from build123d import *

# Parameters (mm, degrees)
F0_R     = 6.35
F0_R_2   = 14.2875
F1_DEPTH = 12.7


with BuildPart() as f1:
    # F0 (on Top) → F1 (new body)
    with BuildSketch(Plane.XY):
        Polygon((-367.050953, -215.623875), (-273.490369, -377.910882), (158.309631, -377.910882), (251.870214, -215.623875), (36.072131, 158.384718), (-151.252869, 158.384718), align=None)
        with Locations((-258.135842, -333.942033)):
            Circle(F0_R, mode=Mode.SUBTRACT)
        with Locations((-289.851294, -278.929488)):
            Circle(F0_R_2, mode=Mode.SUBTRACT)
        with Locations((-321.566746, -223.916943)):
            Circle(F0_R, mode=Mode.SUBTRACT)
        with Locations((142.955103, -333.942033)):
            Circle(F0_R, mode=Mode.SUBTRACT)
        with Locations((174.670555, -278.929488)):
            Circle(F0_R_2, mode=Mode.SUBTRACT)
        with Locations((205.089922, -226.165088)):
            Circle(F0_R, mode=Mode.SUBTRACT)
        with Locations((-121.090369, 122.945368)):
            Circle(F0_R, mode=Mode.SUBTRACT)
        with Locations((-57.590369, 122.945368)):
            Circle(F0_R_2, mode=Mode.SUBTRACT)
        with Locations((5.909631, 122.945368)):
            Circle(F0_R, mode=Mode.SUBTRACT)
    extrude(amount=F1_DEPTH)


solid = f1.part
Source: CAD feature listing. Evaluate the final solid. Frame: model axes, mm. Round coordinates to 2 decimals unless told otherwise and drop trailing zeros. Loops run counter-clockwise (first coordinate to the right, second up) from the corner with the lowest first, then second, coordinate; pieces in that order, holes last. Notation, with made-up numbers: M 21.25,63.25 L 51.25,63.25 A7 ccw 51.25,75.25 Z; hole C 65,-35.5 d2. An arc over 180 degrees is marked long. Answer as CSV lines item,"result".
Q1. Cut plane C-C (y = -49). Return the cut outline in (x, z), plus the area to 3 significant figures.
Verdict:
outline,"M -270.91,0 L 155.73,0 L 155.73,12.7 L -270.91,12.7 Z"
area,"5,420 mm^2"
Q2. Cut plane B-B (x = 52.5). Return the cut outline in (y, z), plus the area to 3 significant figures.
Verdict:
outline,"M -377.91,0 L 129.91,0 L 129.91,12.7 L -377.91,12.7 Z"
area,"6,450 mm^2"
Q3. Cut plane A-A (z = 5.25). Count the separate pieces of the cut face and the enclosed holes in it, plus the area to 3 significant figures.
Verdict:
separate pieces,"1"
enclosed holes,"9"
area,"233,000 mm^2"
Q4. Contact query for flat-ended pins moving along their axis: pin 1 (5 mm diameter, centred on y = 74.5, z = 4, fed in from -X); pin 2 (6 mm diameter, centred on x = -209, z = 11, fed in from +Y); pin 3 (11.5 mm diameter, centred on x = 5.91, y = 122.95, fed in from -Z); pin 4 (3 mm diameter, centred on y = 15.5, z = 7.5, fed in from +X). Output: stop coordinate, or through.
Verdict:
pin 1,"stops at x = -201.1"
pin 2,"stops at y = 63.5"
pin 3,"passes through"
pin 4,"stops at x = 119.38"
Q5. Pull-direction query (X, two-part tool) for faces 1 (the face through (-61, -377.911, 6)), 2 (the face through (-318.153, -218.563, 6.261)), 3 (the face through (-320.926, -295.631, 6.261)); classes: +X half, -X half, draft (parallel to the pull), parting line (faces both ways), or undercut.
Verdict:
face 1,"draft"
face 2,"undercut"
face 3,"-X half"
Q6. Line query: line 1 along Y through (x, z) = (3.5, 3); line 2 along X through (y, z) = (125, 8.25); line 3 along Y through (x, z) = (-281.5, 3.75). Output: solid intervals per line, ascending.
Verdict:
line 1,"y = -377.91 to 117.07, 128.82 to 158.38"
line 2,"x = -170.52 to -127.1, -115.08 to -71.73, -43.45 to -0.1, 11.92 to 55.33"
line 3,"y = -364.02 to -290.52, -267.34 to -67.35"
